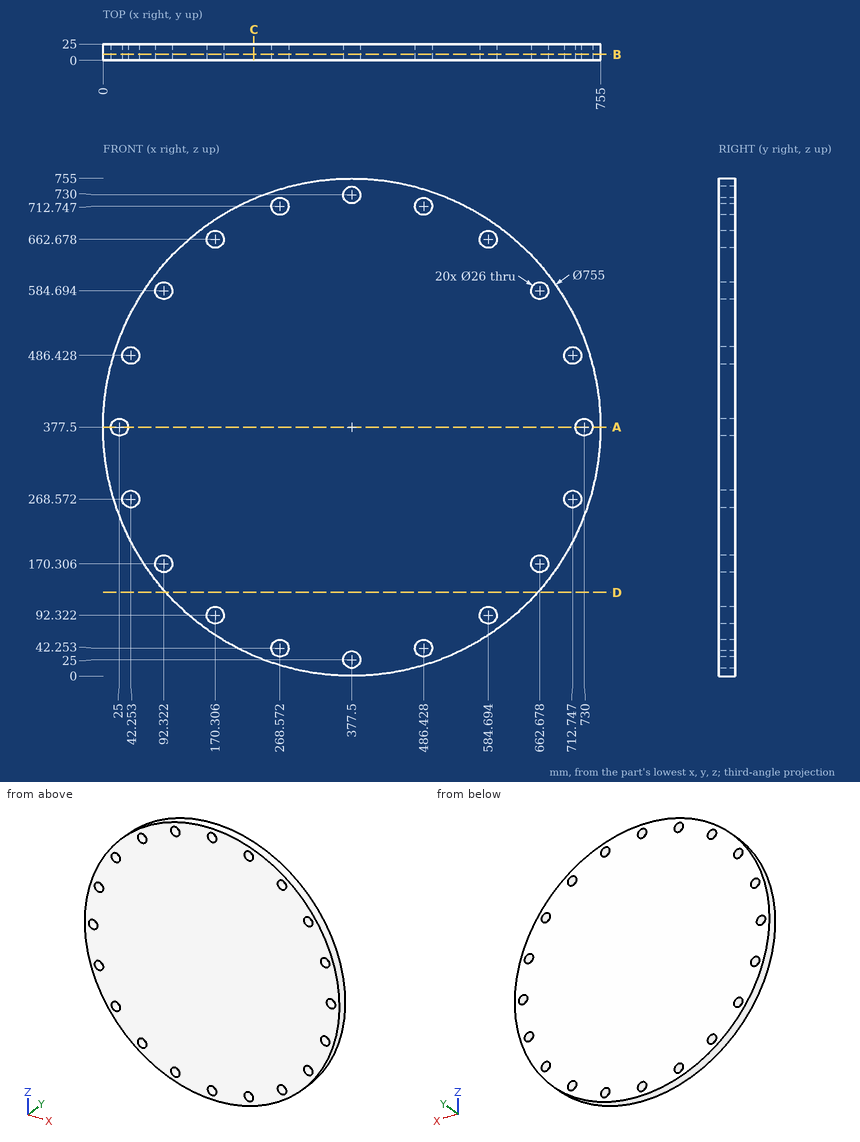
The figure shows three views and two pictorial views of one solid part (mm, origin at its lowest corner). Answer the questions. Coordinates: 2 decimals unless noted, no trailing zeros. Order: outer loops, then holes, each group sorted by start corner. A loop starts at its lowest first (then second) coordinate and runs counter-clockwise, first axis right, second up.
Q1. A cutting plane is placed at D-D, the plane z = 127. Write down the section's boundary in (x, y).
Q2. A cutting plane is placed at C-C, the plane x = 229. Write down the section's boundary in (y, z) (1 decimal), and give its area (3 significant figures).
Q3. Consider line 1 (Z direction, x = 272, y = 15.5); line 2 (Z direction, x = 582, y = 4.5) (1 decimal); line 3 (X direction, y = 9.25, z = 590) (1 decimal). Determine where each line is inside the solid, lowest interval first.
Q4. A cutting plane is placed at A-A, the plane z = 377.5. Write down the section's boundary in (x, y).
Q5. A cutting plane is placed at B-B, the plane y = 9.25. State how many separate pieces and enclosed holes the cut face has, and give its area (3 significant figures).
Q6. Given P1, Ø6, axis at x = 678.5, y = 14.5, coming from the -Z side; P2, Ø2, axis at y = 7.5, z = 648.5, coming from the +X side; P3, Ø12, axis at y = 8.5, z = 109.5, coming from the +X side (1 decimal); P4, Ø12, axis at x = 268, z = 312, coming from the -Y side, each flat-ended and moving along its own axis, determine where each tip first touches the part or whether it passes through.
Answers follow:
1. outline: (95.09, 0) - (659.91, 0) - (659.91, 25) - (95.09, 25) - close
2. outline: (0, 30.4) - (25, 30.4) - (25, 724.6) - (0, 724.6) - close
2. area: 17,400 mm2
3. line 1: z = 15.04 to 29.71, 54.79 to 700.21, 725.29 to 739.96
3. line 2: z = 60.2 to 79.6, 105 to 650, 675.4 to 694.8
3. line 3: x = 65.5 to 80.5, 104.2 to 650.8, 674.5 to 689.5
4. outline: (0, 0) - (12, 0) - (12, 25) - (0, 25) - close; (38, 0) - (717, 0) - (717, 25) - (38, 25) - close; (743, 0) - (755, 0) - (755, 25) - (743, 25) - close
5. separate pieces: 1
5. enclosed holes: 20
5. area: 437,000 mm2
6. P1: stops at z = 145.76
6. P2: stops at x = 641.33
6. P3: stops at x = 649.3
6. P4: stops at y = 0
